```python
from build123d import *

# Parameters (mm, degrees)
BOSS_EXTRUDE1_DEPTH = 3
SKETCH4_W           = 3
SKETCH4_H           = 10
SKETCH4_H_2         = 15.175339059
BOSS_EXTRUDE3_DEPTH = 3
CUT_EXTRUDE1_DEPTH  = 10
SKETCH6_W           = 3
SKETCH6_H           = 12
SKETCH6_H_2         = 18
BOSS_EXTRUDE4_DEPTH = 3
CUT_EXTRUDE2_DEPTH  = 3


with BuildPart() as part:
    # Sketch2 → Boss-Extrude1 (new body)
    with BuildSketch(Plane(origin=(0, 0, 0), x_dir=(0, 0, -1), z_dir=(1, 0, 0))):
        Polygon((0, 0), (0, 35.355339059), (35.355339059, 0), align=None)
    extrude(amount=BOSS_EXTRUDE1_DEPTH)

    # Sketch4 → Boss-Extrude3 (add)
    with BuildSketch(Plane.XZ):
        with Locations((1.5, -5)):
            Rectangle(SKETCH4_W, SKETCH4_H)
        with Locations((1.5, -27.76766953)):
            Rectangle(SKETCH4_W, SKETCH4_H_2)
    extrude(amount=BOSS_EXTRUDE3_DEPTH)

    # Sketch5 → Cut-Extrude1 (cut)
    with BuildSketch(Plane(origin=(3, 0, 0), x_dir=(0, 0, -1), z_dir=(1, 0, 0))):
        Polygon((13.45, 0), (13.45, 2.9), (12.05, 2.9), (12.05, 5.6), (13.45, 5.6), (13.45, 7.3), (16.55, 7.3), (16.55, 5.6), (17.95, 5.6), (17.95, 2.9), (16.55, 2.9), (16.55, 0), align=None)
    extrude(amount=-CUT_EXTRUDE1_DEPTH, mode=Mode.SUBTRACT)

    # Sketch6 → Boss-Extrude4 (add)
    with BuildSketch(Plane(origin=(0, 17.67766953, -17.67766953), x_dir=(1, 0, 0), z_dir=(0, 0.7071067811865515, -0.7071067811865437))):
        with Locations((1.5, -19)):
            Rectangle(SKETCH6_W, SKETCH6_H)
        with Locations((1.5, 16)):
            Rectangle(SKETCH6_W, SKETCH6_H_2)
    extrude(amount=BOSS_EXTRUDE4_DEPTH)

    # Sketch7 → Cut-Extrude2 (cut)
    with BuildSketch(Plane(origin=(3, 0, 0), x_dir=(0, 0, -1), z_dir=(1, 0, 0))):
        Polygon((14.919953083, 20.435385976), (12.869343418, 18.384776311), (13.859292911, 17.394826817), (11.950104602, 15.485638508), (10.960155108, 16.475588002), (9.75807358, 15.273506474), (7.566042559, 17.465537495), (8.768124087, 18.667619023), (7.778174593, 19.657568517), (9.687362902, 21.566756826), (10.677312396, 20.576807333), (12.727922061, 22.627416998), align=None)
    extrude(amount=-CUT_EXTRUDE2_DEPTH, mode=Mode.SUBTRACT)


solid = part.part
```
Here's how the part is built. I have some questions about the finished solid (model axes, mm). A direction names the side the tool comes from. Give positions to 0.01 mm unless a question says otherwise; leave off trailing zeros. Order: outer loops, then holes, each group sorted by start corner. A loop starts at its lowest first (then second) coordinate and runs counter-clockwise, first axis right, second up. Notation, with made-up numbers: (13.25, 0) - (42.25, 0) arc R18 cw to (42.25, 28) - close; hole circle Ø3 at (30, -9.75). An arc over 180 degrees is marked (long way). Answer as a JSON object with one key per item and string values. Group by question number.
Item 1: If we section it at B-B on y = 25.5: Please give me the cut outline in (x, z).
Item 2: Please list where these lines run through material, in increasing order: probe 1 along Z at (x, y) = (0.5, 16); probe 2 along Y at (x, z) = (1.1, -34); probe 3 along Y at (x, z) = (0.9, -9).
Item 3: Which directions (+Z, -Z, +X, -X, +Y, -Y) give clear straight access to the entire face, cutting with the end or side of a thin tool? Please do faces 5 (the flat face through (1.5, 13.8, -23.7)), 6 (the flat face through (1.5, 8.4, -31.2)), 7 (the flat face through (1.52, 16.35, -8.68)), 8 (the flat face through (2, 6, -13.45)).
Item 4: If we section it at C-C on z = -25.5: Please give me the cut outline in (x, y).
Item 5: If we mould it in two halves opening along Z, with no side actions, what happens to faces 1 (the flat face through (2, 7.3, -15)), 2 (the flat face through (1.479, 27.916, -9.531)), 3 (the flat face through (1.521, 19.424, -13.909)), 4 (the flat face through (1, -3, -5))? For each: pulls with the +Z half, pulls with the -Z half, needs draft (parallel to the pull), parting line crosses it, or undercut.
Item 6: For P1, Ø1.5, axis at x = 1.5, z = -15, coming from the -Y side; P2, Ø1.5, axis at x = 1.5, z = -12, coming from the -Y side; P3, Ø1.4, axis at x = 1.5, y = 6.5, coming from the -Z side, each with a flat end and sliding along its axis, tell me the tip position at first contact or that it passes through.
Item 7: If we section it at A-A on z = -17: Please give me the cut outline in (x, y), and give its area (3 significant figures).
Result set:
{
 "1": {"outline": "(0, -9.86) - (3, -9.86) - (3, 0) - (0, 0) - close"},
 "2": {"probe 1": "-19.36 to -12.46, -11.44 to -10.48, -9.03 to 0", "probe 2": "-3 to 5.6", "probe 3": "-3 to 16.03, 20.88 to 26.36, 27.38 to 30.6"},
 "3": {"face 5": "+X, -X, +Y", "face 6": "-Z, +X, -X, +Y", "face 7": "+X, -X", "face 8": "+X, -X, -Y"},
 "4": {"outline": "(0, -3) - (3, -3) - (3, 14.1) - (0, 14.1) - close"},
 "5": {"face 1": "undercut", "face 2": "pulls with the -Z half", "face 3": "undercut", "face 4": "needs draft"},
 "6": {"P1": "y = 7.3", "P2": "y = 0", "P3": "z = -33.8"},
 "7": {"outline": "(0, 0) - (3, 0) - (3, 2.9) - (0, 2.9) - close; (0, 5.6) - (3, 5.6) - (3, 18.36) - (0, 18.36) - close", "area": "47.0 mm²"}
}
